The model under review builds one solid part; all positions refer to its coordinate system, in mm. A direction names the side the tool comes from. Round coordinates to 2 decimals unless told otherwise and drop trailing zeros. Write each loop counter-clockwise with the first axis right and the second up, starting at its lowest first coordinate (ties: lowest second). Pieces come first, ordered by that corner, then holes. Notation, with made-up numbers: (-21, 83) -> (5, 83) arc R29 cw to (5, 115) -> close; hole circle Ø3 at (-22, -6.75). An arc over 180 degrees is marked (long way). Return JSON: item names as keys, results as strings. Group by question number.
1. Take a section at C-C, the plane x = 9.5. Write out the cut boundary in (y, z).
2. Clearance check with flat-ended pins moving along their axes: P1, Ø1, axis at x = 36.5, z = 1, coming from the -Y side; P2, Ø3, axis at x = 4, y = -2.5, coming from the -Z side; P3, Ø1, axis at x = 39, z = 1, coming from the +Y side. State where each tip first meets the part, or that it passes through.
3. Tool access review of faces 4 (the cylindrical face through (-5.1, 7.14, 1.01)), 5 (the flat face through (-6, 0, 1)), 6 (the flat face through (33, 5, 1)), 7 (the flat face through (33, -5, 1)), 8 (the flat face through (2, 0, 1)): name each direction out of +Z, -Z, +X, -X, +Y, -Y from which nothing blocks a thin tool from reaching the whole face with its end or side.
4. Take a section at B-B, the plane x = 53. Write out the cut boundary in (y, z), then the cut area to 3 significant figures.
5. Mouldability with a two-part tool opening along X and no side actions: class faces 1 (the cylindrical face through (59.333, -4.406, 0.986)), 2 (the cylindrical face through (0, -5, 1)), 3 (the flat face through (29, 0, 0)) as pulls with the +X half, pulls with the -X half, needs draft (parallel to the pull), parting line crosses it, or undercut.
6. For line 1 along Y through (x, z) = (0, 1); line 2 along Y through (x, z) = (43.5, 0.85); line 3 along X through (y, z) = (0.75, 0.75), list the stretches that pass through material, from the lowest coordinate up. Write a range as from..to.
7. Take a section at A-A, the plane z = 1.35. Write out the cut boundary in (x, y).
Autodesk Inventor part; units mm, degrees
ref_plane "YZ Plane" through (0, 0, 0) normal (1, 0, 0) x (0, 1, 0)
ref_plane "XZ Plane" through (0, 0, 0) normal (0, 1, 0) x (-1, 0, 0)
ref_plane "XY Plane" through (0, 0, 0) normal (0, 0, 1) x (1, 0, 0)
sketch "スケッチ1" plane through (0, 0, 0) normal (0, 0, 1) x (1, 0, 0)
  line L0 (0, 3) -> (0, -3) construction
  line L1 (-2, 3) -> (-2, -3)
  line L2 (2, -3) -> (2, 3)
  arc A0 (2, 3) -> (-2, 3) centre (0, 3) ccw
  arc A1 (-2, -3) -> (2, -3) centre (0, -3) ccw
  arc A2 (64.2706, 2.7176) -> (54, 5) centre (54, -19.25) ccw
  line L3 (54, 5) -> (12, 5)
  line L4 (-6, 8) -> (0, 8)
  arc A3 (6, 6.5) -> (0, 8) centre (0, -4.75) ccw
  arc A4 (6, 6.5) -> (12, 5) centre (12, 17.75) ccw
  line L5 (-6, 8) -> (-6, 0)
  line L6 (-6, 0) -> (66, 0) construction
  arc A5 (66, 0) -> (64.2706, 2.7176) centre (63, 0) ccw
  arc A6 (54, -5) -> (64.2706, -2.7176) centre (54, 19.25) ccw
  line L7 (54, -5) -> (12, -5)
  line L8 (-6, -8) -> (0, -8)
  arc A7 (12, -5) -> (6, -6.5) centre (12, -17.75) ccw
  line L9 (-6, -8) -> (-6, 0)
  arc A8 (64.2706, -2.7176) -> (66, 0) centre (63, 0) ccw
  arc A9 (0, -8) -> (6, -6.5) centre (0, 4.75) ccw
  point P0 (0, 0)
  point P1 (0, 0)
  point P2 (0, 5)
  point P3 (0, -5)
  dimension "d0" = 4
  dimension "d1" = 10
  dimension "d2" = 8
  dimension "d3" = 6
  dimension "d4" = 0
  dimension "d5" = 5
  dimension "d6" = 12
  dimension "d7" = 6
  dimension "d8" = 72
  dimension "d9" = 3
  dimension "d10" = 9
extrude "押し出し1" add sketch "スケッチ1" along normal blind 2
fillet "フィレット1" radius 3 2 edges at (-6, 8, 1) (-6, -8, 1)
properties part number "fastener_strap"
Output:
{
 "1": {"outline": "(-5.25, 0) -> (5.25, 0) -> (5.25, 2) -> (-5.25, 2) -> close"},
 "2": {"P1": "stops at y = -5", "P2": "stops at z = 0", "P3": "stops at y = 5"},
 "3": {"face 4": "+Z, -Z, -X, +Y", "face 5": "+Z, -Z, -X, +Y, -Y", "face 6": "+Z, -Z, +X, +Y", "face 7": "+Z, -Z, +X, -Y", "face 8": "+Z, -Z"},
 "4": {"outline": "(-5, 0) -> (5, 0) -> (5, 2) -> (-5, 2) -> close", "area": "20.0 mm^2"},
 "5": {"face 1": "pulls with the +X half", "face 2": "undercut", "face 3": "needs draft"},
 "6": {"line 1": "y = -8..-5, 5..8", "line 2": "y = -5..5", "line 3": "x = -6..-2, 2..65.9"},
 "7": {"outline": "(-6, -5) arc R3 ccw to (-3, -8) -> (0, -8) arc R12.75 ccw to (6, -6.5) arc R12.75 cw to (12, -5) -> (54, -5) arc R24.25 ccw to (64.27, -2.72) arc R3 ccw to (66, 0) arc R3 ccw to (64.27, 2.72) arc R24.25 ccw to (54, 5) -> (12, 5) arc R12.75 cw to (6, 6.5) arc R12.75 ccw to (0, 8) -> (-3, 8) arc R3 ccw to (-6, 5) -> close; hole (-2, -3) arc R2 ccw to (2, -3) -> (2, 3) arc R2 ccw to (-2, 3) -> close"}
}
